from build123d import *

# Parameters (mm, degrees)
F1_DEPTH = 9.525
F3_DEPTH = 9.526
F6_DEPTH = 12.7
F7_DEPTH = 12.7
F8_DEPTH = 12.7


with BuildPart() as f1:
    # F0 (on Top) → F1 (new body)
    with BuildSketch(Plane.XY):
        Polygon((-16.5253259897, 63.4753721058), (-41.9253259897, 63.4753721058), (-41.9253259897, -63.5246278942), (53.3246740103, -63.5246278942), (53.3246740103, -38.1246278942), align=None)
    extrude(amount=F1_DEPTH)

    # F2 (on face) → F3 (cut, through all)
    with BuildSketch(Plane.XY.offset(9.525)):
        with BuildLine():
            ThreePointArc((-4.3430600399, 12.1298858759), (-15.7289100643, 16.0767315562), (-22.8753259897, 6.3739530353))
            Line((-22.8753259897, 6.3739530353), (-22.8753259897, -34.3146278942))
            ThreePointArc((-22.8753259897, -34.3146278942), (-19.8995308866, -41.498832791), (-12.7153259897, -44.4746278942))
            Line((-12.7153259897, -44.4746278942), (15.2580733993, -44.4746278942))
            ThreePointArc((15.2580733993, -44.4746278942), (24.2498996226, -39.0446026478), (23.6303393492, -28.5586950536))
            Line((23.6303393492, -28.5586950536), (-4.3430600399, 12.1298858759))
        make_face()
    extrude(amount=-F3_DEPTH, mode=Mode.SUBTRACT)

    # F5 (on face) → F6 (cut)
    with BuildSketch(Plane(origin=(-41.9253259897, 0, 0), x_dir=(0, -1, 0), z_dir=(-1, 0, 0))):
        with BuildLine():
            ThreePointArc((-41.2503721058, 4.7625), (-44.4253721058, 7.9375), (-47.6003721058, 4.7625))
            Line((-47.6003721058, 4.7625), (-41.2503721058, 4.7625))
        make_face()
        with BuildLine():
            ThreePointArc((47.6496278942, 4.7625), (44.4746278942, 7.9375), (41.2996278942, 4.7625))
            Line((41.2996278942, 4.7625), (47.6496278942, 4.7625))
        make_face()
        with BuildLine():
            Line((47.6496278942, 4.7625), (41.2996278942, 4.7625))
            ThreePointArc((41.2996278942, 4.7625), (44.4746278942, 1.5875), (47.6496278942, 4.7625))
        make_face()
        with BuildLine():
            ThreePointArc((3.1996278942, 4.7625), (0.0246278942, 7.9375), (-3.1503721058, 4.7625))
            Line((-3.1503721058, 4.7625), (3.1996278942, 4.7625))
        make_face()
        with BuildLine():
            Line((3.1996278942, 4.7625), (-3.1503721058, 4.7625))
            ThreePointArc((-3.1503721058, 4.7625), (0.0246278942, 1.5875), (3.1996278942, 4.7625))
        make_face()
        with BuildLine():
            Line((-41.2503721058, 4.7625), (-47.6003721058, 4.7625))
            ThreePointArc((-47.6003721058, 4.7625), (-44.4253721058, 1.5875), (-41.2503721058, 4.7625))
        make_face()
    extrude(amount=-F6_DEPTH, mode=Mode.SUBTRACT)

    # F4 (on face) → F7 (cut)
    with BuildSketch(Plane.XZ.offset(63.5246278942)):
        with BuildLine():
            ThreePointArc((-19.7003259897, 4.7625), (-22.8753259897, 7.9375), (-26.0503259897, 4.7625))
            Line((-26.0503259897, 4.7625), (-19.7003259897, 4.7625))
        make_face()
        with BuildLine():
            ThreePointArc((37.4496740103, 4.7625), (34.2746740103, 7.9375), (31.0996740103, 4.7625))
            Line((31.0996740103, 4.7625), (37.4496740103, 4.7625))
        make_face()
        with BuildLine():
            Line((37.4496740103, 4.7625), (31.0996740103, 4.7625))
            ThreePointArc((31.0996740103, 4.7625), (34.2746740103, 1.5875), (37.4496740103, 4.7625))
        make_face()
        with BuildLine():
            ThreePointArc((8.8746740103, 4.7625), (5.6996740103, 7.9375), (2.5246740103, 4.7625))
            Line((2.5246740103, 4.7625), (8.8746740103, 4.7625))
        make_face()
        with BuildLine():
            Line((8.8746740103, 4.7625), (2.5246740103, 4.7625))
            ThreePointArc((2.5246740103, 4.7625), (5.6996740103, 1.5875), (8.8746740103, 4.7625))
        make_face()
        with BuildLine():
            Line((-19.7003259897, 4.7625), (-26.0503259897, 4.7625))
            ThreePointArc((-26.0503259897, 4.7625), (-22.8753259897, 1.5875), (-19.7003259897, 4.7625))
        make_face()
    extrude(amount=-F7_DEPTH, mode=Mode.SUBTRACT)

    # F4 (on face) → F8 (cut)
    with BuildSketch(Plane.XZ.offset(63.5246278942)):
        with BuildLine():
            ThreePointArc((-19.7003259897, 4.7625), (-22.8753259897, 7.9375), (-26.0503259897, 4.7625))
            Line((-26.0503259897, 4.7625), (-19.7003259897, 4.7625))
        make_face()
        with BuildLine():
            ThreePointArc((37.4496740103, 4.7625), (34.2746740103, 7.9375), (31.0996740103, 4.7625))
            Line((31.0996740103, 4.7625), (37.4496740103, 4.7625))
        make_face()
        with BuildLine():
            Line((37.4496740103, 4.7625), (31.0996740103, 4.7625))
            ThreePointArc((31.0996740103, 4.7625), (34.2746740103, 1.5875), (37.4496740103, 4.7625))
        make_face()
        with BuildLine():
            ThreePointArc((8.8746740103, 4.7625), (5.6996740103, 7.9375), (2.5246740103, 4.7625))
            Line((2.5246740103, 4.7625), (8.8746740103, 4.7625))
        make_face()
        with BuildLine():
            Line((8.8746740103, 4.7625), (2.5246740103, 4.7625))
            ThreePointArc((2.5246740103, 4.7625), (5.6996740103, 1.5875), (8.8746740103, 4.7625))
        make_face()
        with BuildLine():
            Line((-19.7003259897, 4.7625), (-26.0503259897, 4.7625))
            ThreePointArc((-26.0503259897, 4.7625), (-22.8753259897, 1.5875), (-19.7003259897, 4.7625))
        make_face()
    extrude(amount=-F8_DEPTH, mode=Mode.SUBTRACT)


solid = f1.part
Could you check a few things on this model? Use its own coordinates, in mm. A direction names the side the tool comes from. Coordinates: 2 decimals unless noted, no trailing zeros. Order: outer loops, then holes, each group sorted by start corner. A loop starts at its lowest first (then second) coordinate and runs counter-clockwise, first axis right, second up. Notation, with made-up numbers: (-15, 49) -> (30, 49) arc R15 ccw to (30, 77) -> close; hole circle Ø1 at (10.25, 84). An arc over 180 degrees is marked (long way). One line per item, written item: value. Start each with the question number.
1) Imagine slicing it at B-B on y = -22. List the corners of the cut face in (x, z) for me (3 decimals).
2) Which directions (+Z, -Z, +X, -X, +Y, -Y) give clear straight access to the entire face, cutting with the end or side of a thin tool? Please do faces 5 (the flat face through (18.89, 11.96, 4.7)), 6 (the flat face through (5, -63.525, 1.5)), 7 (the cylindrical face through (8.04, -57.264, 2.617)), 8 (the flat face through (9.84, -8.5, 4.83)), 9 (the cylindrical face through (-35.664, 41.253, 4.623)).
3) Imagine slicing it at D-D on y = 45. List the corners of the cut face in (x, z) for me (1 decimal).
4) If I drill on L1, parallel to Y at x = -30, z = 3.75; L2, parallel to Y at x = 13.5, z = 9; L3, parallel to X at y = -18, z = 7.25, over which ranges is the centre line in solid material (lowest first)? Write a range as [from, to].
5) We'd pull the mould along Y, two halves only. Please class faces 1 (the flat face through (6, -50.825, 5)), 2 (the cylindrical face through (31.246, -57.264, 3.809)), 3 (the cylindrical face through (-35.664, -41.446, 3.809)), 4 (the flat face through (-29.225, 0, 5)): +Y half, -Y half, draft (parallel to the pull), parting line (faces both ways), or undercut.
6) Imagine slicing it at A-A on y = -54. Count the separate pieces of the cut face and the enclosed holes in it, plus the area to 3 significant figures.
7) I'm going to push flat-ended pins straight in: pin 1 (3 mm diameter, centred on x = 34, z = 5, fed in from -Y); pin 2 (5 mm diameter, centred on y = -0.02, z = 4.76, fed in from -X); pin 3 (4 mm diameter, centred on x = 34.27, z = 4.76, fed in from +Y). Where does each tip first touch, or does it pass through?
Answer list:
1. outline: (-41.925, 0) -> (-22.875, 0) -> (-22.875, 9.525) -> (-41.925, 9.525) -> close; (19.121, 0) -> (42.239, 0) -> (42.239, 9.525) -> (19.121, 9.525) -> close
2. face 5: +Z, -Z, +X, +Y
2. face 6: +Z, -Z, +X, -X, -Y
2. face 7: -Y
2. face 8: +Z, -Z
2. face 9: -X
3. outline: (-41.9, 0) -> (-3.8, 0) -> (-3.8, 9.5) -> (-41.9, 9.5) -> (-41.9, 7.9) -> (-29.2, 7.9) -> (-29.2, 1.6) -> (-41.9, 1.6) -> close
4. L1: y = [-63.52, -47.48], [-41.47, -3.03], [2.98, 41.42], [47.43, 63.48]
4. L2: y = [-63.52, -44.47], [-13.82, 19.8]
4. L3: x = [-41.93, -22.88], [16.37, 39.49]
5. face 1: -Y half
5. face 2: draft
5. face 3: undercut
5. face 4: undercut
6. separate pieces: 1
6. enclosed holes: 3
6. area: 812 mm2
7. pin 1: stops at y = -50.82
7. pin 2: stops at x = -29.23
7. pin 3: stops at y = -7.5
